Check sheet for the modelled part. Datum: model origin and axes. Units: mm. Face numbers are marked on the shaded views. A direction names the side the tool comes from. Give positions to 0.01 mm unless a question says otherwise; leave off trailing zeros. Order: outer loops, then holes, each group sorted by start corner. A loop starts at its lowest first (then second) coordinate and runs counter-clockwise, first axis right, second up.
Item 1: Access from +Z, -Z, +X, -X, +Y, -Y to the whole of each face (thin tool, end or side, straight path). Record for the marked faces 1 and 2.
Item 2: Sectioned sample at B-B on z = 22.5. Record the boundary of the cut face in (x, y).
Item 3: Sectioned sample at C-C on x = -5.5. Record the boundary of the cut face in (y, z).
Item 4: Sectioned sample at A-A on y = 0. Record the boundary of the cut face in (x, z).
Item 5: Gauge pin test, flat ends, axial feed: P1, Ø5, axis at y = -7, z = 45, coming from the +X side; P2, Ø1.5, axis at x = -7, z = 18, coming from the -Y side; P3, Ø8, axis at x = 8, z = 22.5, coming from the -Y side. Record the tip position at first contact, or that the pin passes through.
Item 6: Material ranges on line 1 along Y through (x, z) = (-0.25, 32.5); line 2 along Y through (x, z) = (10.25, 20.5); line 3 along X through (y, z) = (-4.25, 7), recorded low to high.
Item 7: Sectioned sample at D-D on y = 6.5. Record the boundary of the cut face in (x, z).
Autodesk Inventor part; units mm, degrees
ref_plane "YZ Plane" through (0, 0, 0) normal (1, 0, 0) x (0, 1, 0)
ref_plane "XZ Plane" through (0, 0, 0) normal (0, 1, 0) x (-1, 0, 0)
ref_plane "XY Plane" through (0, 0, 0) normal (0, 0, 1) x (1, 0, 0)
sketch "Sketch1" plane through (0, 0, 0) normal (0, 0, 1) x (1, 0, 0)
  circle A0 centre (0, 0) radius 13.5255
  dimension "d0" = 27.051
extrude "Extrusion1" add sketch "Sketch1" along normal blind 54.0766
sketch "Sketch2" plane through (0, 0, 0) normal (1, 0, 0) x (0, 1, 0)
  circle A0 centre (0, 21.742) radius 9.8044
  point P0 (0, 0)
  dimension "d3" = 19.6088
extrude "Extrusion2" add sketch "Sketch2" along normal blind 14.8082
sketch "Sketch3" plane through (14.8082, 0, 21.742) normal (1, 0, 0) x (0, 0, -1)
  circle A0 centre (0, 0) radius 1.5
  point P0 (21.742, 0)
  dimension "d6" = 3
extrude "Extrusion3" cut sketch "Sketch3" against normal blind 14.8082
properties part number "Camera"
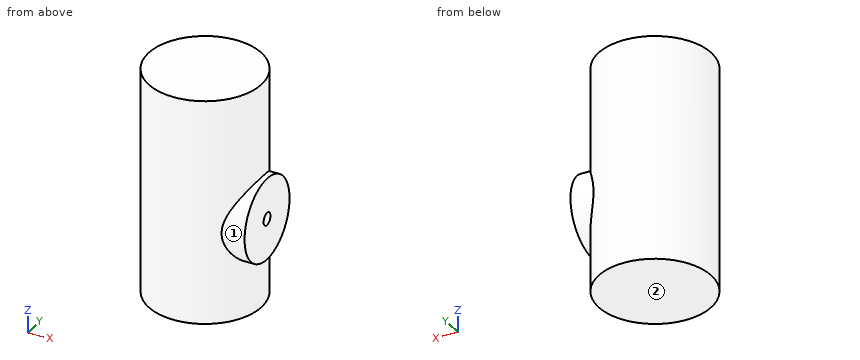
Report:
1. face 1: +X
1. face 2: -Z, +X, -X, +Y, -Y
2. outline: (0, -1.29) - (0, 1.29) - (14.81, 1.29) - (14.81, 9.78) - (9.35, 9.78) arc R13.53 ccw (long way) to (9.35, -9.78) - (14.81, -9.78) - (14.81, -1.29) - close
3. outline: (-12.36, 0) - (12.36, 0) - (12.36, 54.08) - (-12.36, 54.08) - close
4. outline: (-13.53, 0) - (13.53, 0) - (13.53, 11.94) - (14.81, 11.94) - (14.81, 20.24) - (0, 20.24) - (0, 23.24) - (14.81, 23.24) - (14.81, 31.55) - (13.53, 31.55) - (13.53, 54.08) - (-13.53, 54.08) - close
5. P1: stops at x = 12.75
5. P2: stops at y = -11.99
5. P3: stops at y = -12.92
6. line 1: y = -13.52 to 13.52
6. line 2: y = -9.73 to -0.84, 0.84 to 9.73
6. line 3: x = -12.84 to 12.84
7. outline: (-11.86, 0) - (11.86, 0) - (11.86, 14.4) - (14.81, 14.4) - (14.81, 29.08) - (11.86, 29.08) - (11.86, 54.08) - (-11.86, 54.08) - close
